Read the model definition and answer for the solid it produces. Units are mm, in the model's axes. A direction names the side the tool comes from. Coordinates: 2 decimals unless noted, no trailing zeros. Write each loop counter-clockwise with the first axis right and the second up, starting at its lowest first coordinate (ties: lowest second). Pieces come first, ordered by that corner, then holes.
1) The part is cut by section A-A (y = -1.55). Determine the outline of the cut face in (x, z).
2) The part is cut by section D-D (x = 36.25). Determine the outline of the cut face in (y, z), then the cut area to 3 significant figures.
3) The part is cut by section B-B (z = -9.8). Determine the outline of the cut face in (x, y).
4) Determine the mould class of faces 4 (the face through (35.08, -1.25, -9.45)), 5 (the face through (39, -1, -10.969)), 6 (the face through (41.05, -1, -9)), 7 (the face through (38, -1, -10.089)) for opening direction X: +X half, -X half, draft (parallel to the pull), parting line (faces both ways), or undercut.
5) The part is cut by section C-C (z = -9.4). Determine the outline of the cut face in (x, y).
6) Each of these flat-tipped pins is pushed along its axis until it touches: pin 1 Ø1.3 at (x, y) = (38.5, -1.5) entering from +Z; pin 2 Ø1 at (y, z) = (-1, -9) entering from +X. Where does it stop, or does it pass through?
7) Find the intervals of material crossed by line 1 (X direction, y = -1, z = -9.8); line 2 (Z direction, x = 43, y = -0.9); line 3 (X direction, y = -2.3, z = -9.6), in increasing order.
8) Which of the six approach directions +Z, -Z, +X, -X, +Y, -Y give full straight-line access (tool end or side, diameter ignored) to faces 1 (the face through (42, -1, -10.089)), 2 (the face through (39, 0, -10.3)), 3 (the face through (40.015, -1.252, -9.788))?
from build123d import *

# Parameters (mm, degrees)
F0_R     = 0.44
F1_DEPTH = 2.54


with BuildPart() as f1:
    # F0 (on Front) → F1 (new body)
    with BuildSketch(Plane.XZ):
        with BuildLine():
            Line((38.29968, -10.089144), (36.56368, -10.089144))
            ThreePointArc((36.56368, -10.089144), (35.061426, -9.46689), (35.68368, -10.969144))
            Line((35.68368, -10.969144), (40.29968, -10.969144))
            Line((40.29968, -10.969144), (43.32968, -10.969144))
            Line((43.32968, -10.969144), (43.32968, -10.089144))
            Line((43.32968, -10.089144), (41.04968, -10.089144))
            Line((41.04968, -10.089144), (41.04968, -8.919144))
            Line((41.04968, -8.919144), (41.04968, -8.819144))
            ThreePointArc((41.04968, -8.819144), (41.020391, -8.748433), (40.94968, -8.719144))
            Line((40.94968, -8.719144), (40.29968, -8.719144))
            Line((40.29968, -8.719144), (40.29968, -9.089144))
            ThreePointArc((40.29968, -9.089144), (40.006787, -9.79625), (39.29968, -10.089144))
            Line((39.29968, -10.089144), (38.29968, -10.089144))
        make_face()
        with Locations((35.68368, -10.089144)):
            Circle(F0_R, mode=Mode.SUBTRACT)
    extrude(amount=F1_DEPTH)


solid = f1.part
Reported:
1. outline: (35.68, -10.97) - (43.33, -10.97) - (43.33, -10.09) - (41.05, -10.09) - (41.05, -8.82) arc R0.1 ccw to (40.95, -8.72) - (40.3, -8.72) - (40.3, -9.09) arc R1 cw to (39.3, -10.09) - (36.56, -10.09) arc R0.88 ccw (long way) to start; hole circle Ø0.88 at (35.68, -10.09)
2. outline: (-2.54, -10.97) - (0, -10.97) - (0, -9.42) - (-2.54, -9.42) - close
2. area: 3.95 mm2
3. outline: (34.85, -2.54) - (35.35, -2.54) - (35.35, 0) - (34.85, 0) - close; (36.02, -2.54) - (36.51, -2.54) - (36.51, 0) - (36.02, 0) - close; (40, -2.54) - (41.05, -2.54) - (41.05, 0) - (40, 0) - close
4. face 4: undercut
4. face 5: draft
4. face 6: +X half
4. face 7: undercut
5. outline: (35.14, -2.54) - (36.23, -2.54) - (36.23, 0) - (35.14, 0) - close; (40.25, -2.54) - (41.05, -2.54) - (41.05, 0) - (40.25, 0) - close
6. pin 1: stops at z = -10.09
6. pin 2: stops at x = 41.05
7. line 1: x = 34.85 to 35.35, 36.02 to 36.51, 40 to 41.05
7. line 2: z = -10.97 to -10.09
7. line 3: x = 34.95 to 36.42, 40.16 to 41.05
8. face 1: +Z, +X, +Y, -Y
8. face 2: +Z, -Z, +X, -X, +Y
8. face 3: +Z, +Y, -Y
